The listing builds one solid part. Answer for the finished solid, in the listing's coordinates (mm). A direction names the side the tool comes from. Round coordinates to 2 decimals unless told otherwise and drop trailing zeros. Write each loop counter-clockwise with the first axis right and the second up, starting at its lowest first coordinate (ties: lowest second). Pieces come first, ordered by that corner, then holes. Notation, with made-up numbers: (-4.5, 11) - (28.5, 11) arc R18 ccw to (28.5, 31) - close; hole circle Ø1 at (-14.75, 78.5). An arc over 180 degrees is marked (long way). Use a Markdown table: item, result. Add a question column.
1) A tool of negligible diameter and unlimited length cuts with its end or side. For faces 1 (the flat face through (-70, 5, -6)), 2 (the cylindrical face through (62.36, 0.585, -2.636)), 3 (the flat face through (-25, 0.1, 10.2)), 4 (the flat face through (67.5, 0, 6)), 5 (the flat face through (70, 5, -6)), from which of +Z, -Z, +X, -X, +Y, -Y can it reach the whole face along a straight path? Write none if from no direction.
2) Find the intervals of material crossed by probe 1 along Z at (x, y) = (-57.25, 0); probe 2 along X at (y, z) = (9, -4.5), in increasing order. Write a range as from..to.
3) Determine the mould class of faces 6 (the cylindrical face through (0.35, -2.17, -9.76)), 7 (the flat face through (70, -5, -6)), 8 (the cylindrical face through (-62.36, -0.585, -2.636)), 9 (the cylindrical face through (70, 0, 5)) for opening direction Z: +Z half, -Z half, draft (parallel to the pull), parting line (faces both ways), or undercut.
4) A cutting plane is placed at D-D (x = 7). Give the vertices of the cut face in (y, z).
5) A cutting plane is placed at C-C (y = 7.5). Give the vertices of the cut face in (x, z).
6) Each of these flat-tipped pins is pushed along its axis until it touches: P1, Ø7, axis at y = 4, z = 5.5, coming from the +X side; P2, Ø6, axis at x = -45, z = -5.5, coming from the -Y side; P3, Ø10, axis at x = 2, y = 8.5, coming from the -Z side; P4, Ø5.5, axis at x = -69.5, z = -8.5, coming from the -Y side. Where does it stop, or does it pass through?
7) A cutting plane is placed at A-A (z = -8.5). Give the vertices of the cut face in (x, y), then the cut area to 3 significant figures.
8) A cutting plane is placed at B-B (x = 35). Give the vertices of the cut face in (y, z).
```python
from build123d import *

# Parameters (mm, degrees)
F0_R      = 10
F1_DEPTH  = 25
F2_R      = 12.5
F3_DEPTH  = 42.5
F4_R      = 12.5
F5_DEPTH  = 42.5
F7_DEPTH  = 5
F9_D      = 5.4
F9_DEPTH  = 20
F9_TIP    = 1.6223236714
F11_DEPTH = 5
F13_D     = 5.4
F13_DEPTH = 20
F13_TIP   = 1.6223236714


with BuildPart() as f1:
    # F0 (on Right) → F1 (new body, symmetric)
    with BuildSketch(Plane.YZ):
        Circle(F0_R)
    extrude(amount=F1_DEPTH, both=True)

    # F2 (on face) → F3 (join)
    with BuildSketch(Plane.YZ.offset(25)):
        Circle(F2_R)
    extrude(amount=F3_DEPTH)

    # F4 (on face) → F5 (join)
    with BuildSketch(Plane(origin=(-25, 0, 0), x_dir=(0, -1, 0), z_dir=(-1, 0, 0))):
        Circle(F4_R)
    extrude(amount=F5_DEPTH)

    # F6 (on face) → F7 (join)
    with BuildSketch(Plane.YZ.offset(67.5)):
        with BuildLine():
            Line((5, -11.4564392374), (5, 0))
            ThreePointArc((5, 0), (0, -5), (-5, 0))
            Line((-5, 0), (-5, -11.4564392374))
            ThreePointArc((-5, -11.4564392374), (0, -12.5), (5, -11.4564392374))
        make_face()
        with BuildLine():
            ThreePointArc((-5, 0), (0, -5), (5, 0))
            ThreePointArc((5, 0), (0, 5), (-5, 0))
        make_face()
    extrude(amount=F7_DEPTH)

    # F9
    with Locations(Plane.YZ.offset(72.5)):
        with Locations((0, 0)):
            Hole(F9_D / 2, depth=F9_DEPTH)
            with Locations((0, 0, -(F9_DEPTH + F9_TIP / 2))):  # 118° drill point
                Cone(0, F9_D / 2, F9_TIP, mode=Mode.SUBTRACT)

    # F10 (on face) → F11 (join)
    with BuildSketch(Plane(origin=(-67.5, 0, 0), x_dir=(0, -1, 0), z_dir=(-1, 0, 0))):
        with BuildLine():
            ThreePointArc((-5, 0), (0, -5), (5, 0))
            ThreePointArc((5, 0), (0, 5), (-5, 0))
        make_face()
        with BuildLine():
            Line((5, -11.4564392374), (5, 0))
            ThreePointArc((5, 0), (0, -5), (-5, 0))
            Line((-5, 0), (-5, -11.4564392374))
            ThreePointArc((-5, -11.4564392374), (0, -12.5), (5, -11.4564392374))
        make_face()
    extrude(amount=F11_DEPTH)

    # F13
    with Locations(Plane(origin=(-72.5, 0, 0), x_dir=(0, -1, 0), z_dir=(-1, 0, 0))):
        with Locations((0, 0)):
            Hole(F13_D / 2, depth=F13_DEPTH)
            with Locations((0, 0, -(F13_DEPTH + F13_TIP / 2))):  # 118° drill point
                Cone(0, F13_D / 2, F13_TIP, mode=Mode.SUBTRACT)


solid = f1.part
```
Entries:
| question | item | result |
|---|---|---|
| 1 | face 1 | +Z, -Z, -X, +Y |
| 1 | face 2 | +X |
| 1 | face 3 | none |
| 1 | face 4 | +Z, +X |
| 1 | face 5 | +Z, -Z, +X, +Y |
| 2 | probe 1 | z = -12.5..-2.7, 2.7..12.5 |
| 2 | probe 2 | x = -67.5..-25, 25..67.5 |
| 3 | face 6 | parting line |
| 3 | face 7 | draft |
| 3 | face 8 | undercut |
| 3 | face 9 | +Z half |
| 4 | outline | circle Ø20 at (0, 0) |
| 5 | outline | (-67.5, -10) - (-25, -10) - (-25, -6.61) - (25, -6.61) - (25, -10) - (67.5, -10) - (67.5, 10) - (25, 10) - (25, 6.61) - (-25, 6.61) - (-25, 10) - (-67.5, 10) - close |
| 6 | P1 | stops at x = 72.5 |
| 6 | P2 | stops at y = -12.25 |
| 6 | P3 | stops at z = -9.37 |
| 6 | P4 | stops at y = -10.61 |
| 7 | outline | (-72.5, -5) - (-67.5, -5) - (-67.5, -9.17) - (-25, -9.17) - (-25, -5.27) - (25, -5.27) - (25, -9.17) - (67.5, -9.17) - (67.5, -5) - (72.5, -5) - (72.5, 5) - (67.5, 5) - (67.5, 9.17) - (25, 9.17) - (25, 5.27) - (-25, 5.27) - (-25, 9.17) - (-67.5, 9.17) - (-67.5, 5) - (-72.5, 5) - close |
| 7 | area | 2,180 mm² |
| 8 | outline | circle Ø25 at (0, 0) |
